```python
from build123d import *

# Parameters (mm, degrees)
F1_DEPTH      = 15.08125
F1_DEPTH_BACK = 15.08125
F2_R          = 63.5
F3_R          = 22.225
F4_R          = 12.7


with BuildPart() as f1:
    # F0 (on Right) → F1 (new body, two sides)
    with BuildSketch(Plane.YZ) as f1_sk:
        Polygon((0, 14.2875), (0, 0), (206.375, 0), (206.375, 30.48), (325.4375, 30.48), (325.4375, 0), (428.625, 0), (428.625, 30.48), (547.6875, 30.48), (547.6875, 0), (609.6, 0), (609.6, 38.1), (584.2, 51.60542), (547.6875, 63.5), (206.375, 63.5), (25.4, 25.06916), align=None)
    extrude(amount=F1_DEPTH)
    extrude(f1_sk.sketch, amount=-F1_DEPTH_BACK)

    # F2
    f2_edges = [f1.edges().sort_by_distance(p)[0] for p in [
        (0, 25.4, 25.06916),
        (0, 206.375, 63.5),
        (0, 547.6875, 63.5),
        (0, 584.2, 51.60542),
    ]]
    fillet(f2_edges, radius=F2_R)

    # F3
    f3_edges = [f1.edges().sort_by_distance(p)[0] for p in [
        (0, 206.375, 30.48),
        (0, 325.4375, 30.48),
        (0, 428.625, 30.48),
        (0, 547.6875, 30.48),
    ]]
    fillet(f3_edges, radius=F3_R)

    # F4
    f4_edges = [f1.edges().sort_by_distance(p)[0] for p in [
        (15.08125, 265.90625, 30.48),
        (-15.08125, 265.90625, 30.48),
        (15.08125, 488.15625, 30.48),
        (-15.08125, 488.15625, 30.48),
        (15.08125, 375.324025, 63.5),
        (-15.08125, 375.324025, 63.5),
    ]]
    fillet(f4_edges, radius=F4_R)


solid = f1.part
```
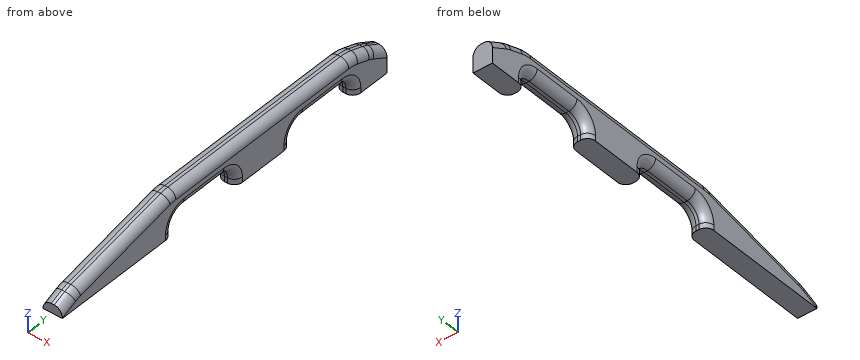
Source: CAD feature listing. Evaluate the final solid. Frame: model axes, mm. Round coordinates to 2 decimals unless told otherwise and drop trailing zeros. Order: outer loops, then holes, each group sorted by start corner. A loop starts at its lowest first (then second) coordinate and runs counter-clockwise, first axis right, second up. Notation, with made-up numbers: (-24.5, 53.25) -> (-16.5, 53.25) arc R30 ccw to (-16.5, 82.25) -> close; hole circle Ø7 at (59.25, -20). An arc over 180 degrees is marked (long way). One line per item, written item: value. Start each with the question number.
Q1. Pin query (flat end, axial travel): pin 1 (5 mm diameter, centred on y = 249.5, z = 56, fed in from +X); pin 2 (4 mm diameter, centred on x = 0.5, y = 250.5, fed in from -Z); pin 3 (8 mm diameter, centred on y = 534, z = 37.5, fed in from +X). Return the tip coordinate at first contact, or that it passes through.
Q2. Material intervals for probe 1 along Y at (x, z) = (3, 8); probe 2 along Y at (x, z) = (3, 9); probe 3 along Z at (x, y) = (7.5, 464.5), sorted ascending.
Q3. Section query A-A (y = 457.5). Return the cut outline in (x, z), plus the area to 3 significant figures.
Findings below:
1. pin 1: x = 14.79
1. pin 2: z = 30.48
1. pin 3: x = 15.07
2. probe 1: 0 to 206.36, 325.45 to 428.61, 547.7 to 609.6
2. probe 2: 0 to 206.37, 325.44 to 428.62, 547.69 to 609.6
2. probe 3: 31.56 to 62.42
3. outline: (-15.08, 43.18) arc R12.7 ccw to (-2.38, 30.48) -> (2.38, 30.48) arc R12.7 ccw to (15.08, 43.18) -> (15.08, 50.8) arc R12.7 ccw to (2.38, 63.5) -> (-2.38, 63.5) arc R12.7 ccw to (-15.08, 50.8) -> close
3. area: 858 mm²
